```python
from build123d import *

# Parameters (mm, degrees)
BOX_W           = 42
BOX_H           = 42
BOX_DEPTH       = 5
SKETCH_R        = 2.75
POCKET_DEPTH    = 2.5
SKETCH001_R     = 1.55
POCKET001_DEPTH = 5
SKETCH002_R     = 2.75
POCKET002_DEPTH = 2.5
SKETCH003_R     = 1.55
POCKET003_DEPTH = 5
CHAMFER_SIZE    = 2
CHAMFER001_SIZE = 2
CHAMFER002_SIZE = 2
CHAMFER003_SIZE = 2
SKETCH004_W     = 16
SKETCH004_H     = 2.5
PAD_DEPTH       = 20
PAD001_DEPTH    = 2
PAD002_DEPTH    = 2
SKETCH007_R     = 1.55
POCKET004_DEPTH = 5
SKETCH008_W     = 20
SKETCH008_H     = 20
POCKET005_DEPTH = 1
SKETCH010_R     = 2.85
SKETCH010_R_2   = 1.75
POCKET006_DEPTH = 2.5
SKETCH011_R     = 1.75
SKETCH011_R_2   = 2.85
POCKET007_DEPTH = 2.5
SKETCH012_R     = 1.75
POCKET008_DEPTH = 5


with BuildPart() as part:
    # Box → Box (new body)
    with BuildSketch(Plane(origin=(-21, -21, 0), x_dir=(1, 0, 0), z_dir=(0, 0, 1))):
        with Locations((21, 21)):
            Rectangle(BOX_W, BOX_H)
    extrude(amount=BOX_DEPTH)

    # Sketch → Pocket (cut)
    with BuildSketch(Plane(origin=(-21, -21, 5), x_dir=(1, 0, 0), z_dir=(0, 0, 1))):
        with Locations((5.5, 5.5)):
            Circle(SKETCH_R)
        with Locations((36.5, 5.5)):
            Circle(SKETCH_R)
        with Locations((36.5, 36.5)):
            Circle(SKETCH_R)
        with Locations((5.5, 36.5)):
            Circle(SKETCH_R)
    extrude(amount=-POCKET_DEPTH, mode=Mode.SUBTRACT)

    # Sketch001 → Pocket001 (cut)
    with BuildSketch(Plane(origin=(-21, -21, 0), x_dir=(1, 0, 0), z_dir=(0, 0, -1))):
        with Locations((5.5, -5.5)):
            Circle(SKETCH001_R)
        with Locations((36.5, -5.5)):
            Circle(SKETCH001_R)
        with Locations((36.5, -36.5)):
            Circle(SKETCH001_R)
        with Locations((5.5, -36.5)):
            Circle(SKETCH001_R)
    extrude(amount=-POCKET001_DEPTH, mode=Mode.SUBTRACT)

    # Sketch002 → Pocket002 (cut)
    with BuildSketch(Plane(origin=(-21, -21, 0), x_dir=(1, 0, 0), z_dir=(0, 0, -1))):
        with Locations((6, -21)):
            Circle(SKETCH002_R)
        with Locations((36, -21)):
            Circle(SKETCH002_R)
    extrude(amount=-POCKET002_DEPTH, mode=Mode.SUBTRACT)

    # Sketch003 → Pocket003 (cut)
    with BuildSketch(Plane(origin=(-21, -21, 5), x_dir=(1, 0, 0), z_dir=(0, 0, 1))):
        with Locations((6, 21)):
            Circle(SKETCH003_R)
        with Locations((36, 21)):
            Circle(SKETCH003_R)
    extrude(amount=-POCKET003_DEPTH, mode=Mode.SUBTRACT)

    # Chamfer
    chamfer_edges = [part.edges().sort_by_distance(p)[0] for p in [
        (-21, -21, 2.5),
    ]]
    chamfer(chamfer_edges, length=CHAMFER_SIZE)

    # Chamfer001
    chamfer001_edges = [part.edges().sort_by_distance(p)[0] for p in [
        (-21, 21, 2.5),
    ]]
    chamfer(chamfer001_edges, length=CHAMFER001_SIZE)

    # Chamfer002
    chamfer002_edges = [part.edges().sort_by_distance(p)[0] for p in [
        (21, 21, 2.5),
    ]]
    chamfer(chamfer002_edges, length=CHAMFER002_SIZE)

    # Chamfer003
    chamfer003_edges = [part.edges().sort_by_distance(p)[0] for p in [
        (21, -21, 2.5),
    ]]
    chamfer(chamfer003_edges, length=CHAMFER003_SIZE)

    # Sketch004 → Pad (new body)
    with BuildSketch(Plane(origin=(-21, -21, 5), x_dir=(1, 0, 0), z_dir=(0, 0, 1))):
        with Locations((21, 31.25)):
            Rectangle(SKETCH004_W, SKETCH004_H)
    extrude(amount=PAD_DEPTH)

    # Sketch005 → Pad001 (new body)
    with BuildSketch(Plane(origin=(-8, -21, 0), x_dir=(0, -1, 0), z_dir=(-1, 0, 0))):
        Polygon((-30, 25), (-32.5, 25), (-41.94515, 5), (-30, 5), align=None)
    extrude(amount=PAD001_DEPTH)

    # Sketch006 → Pad002 (new body)
    with BuildSketch(Plane(origin=(8, -21, 0), x_dir=(0, 1, 0), z_dir=(1, 0, 0))):
        Polygon((30, 25), (32.5, 25), (42, 5), (30, 5), align=None)
    extrude(amount=PAD002_DEPTH)

    # Sketch007 → Pocket004 (cut)
    with BuildSketch(Plane(origin=(-21, 11.5, 0), x_dir=(-1, 0, 0), z_dir=(0, 1, 0))):
        with Locations((-21, 15)):
            Circle(SKETCH007_R)
    extrude(amount=-POCKET004_DEPTH, mode=Mode.SUBTRACT)

    # Sketch008 → Pocket005 (cut)
    with BuildSketch(Plane(origin=(-21, 9, 0), x_dir=(1, 0, 0), z_dir=(0, -1, 0))):
        with Locations((21, 15)):
            Rectangle(SKETCH008_W, SKETCH008_H)
    extrude(amount=-POCKET005_DEPTH, mode=Mode.SUBTRACT)

    # Sketch010 → Pocket006 (cut)
    with BuildSketch(Plane(origin=(-21, -21, 5), x_dir=(1, 0, 0), z_dir=(0, 0, 1))):
        with Locations((5.5, 36.5)):
            Circle(SKETCH010_R)
        with Locations((5.5, 5.5)):
            Circle(SKETCH010_R)
        with Locations((36.5, 5.5)):
            Circle(SKETCH010_R)
        with Locations((36, 21)):
            Circle(SKETCH010_R_2)
        with Locations((36.5, 36.5)):
            Circle(SKETCH010_R)
        with Locations((6, 21)):
            Circle(SKETCH010_R_2)
    extrude(amount=-POCKET006_DEPTH, mode=Mode.SUBTRACT)

    # Sketch011 → Pocket007 (cut)
    with BuildSketch(Plane(origin=(-21, -21, 0), x_dir=(1, 0, 0), z_dir=(0, 0, -1))):
        with Locations((5.5, -5.5)):
            Circle(SKETCH011_R)
        with Locations((36.5, -5.5)):
            Circle(SKETCH011_R)
        with Locations((6, -21)):
            Circle(SKETCH011_R_2)
        with Locations((36, -21)):
            Circle(SKETCH011_R_2)
        with Locations((36.5, -36.5)):
            Circle(SKETCH011_R)
        with Locations((5.5, -36.5)):
            Circle(SKETCH011_R)
    extrude(amount=-POCKET007_DEPTH, mode=Mode.SUBTRACT)

    # Sketch012 → Pocket008 (cut)
    with BuildSketch(Plane(origin=(-21, 10, 0), x_dir=(1, 0, 0), z_dir=(0, -1, 0))):
        with Locations((21, 15)):
            Circle(SKETCH012_R)
    extrude(amount=-POCKET008_DEPTH, mode=Mode.SUBTRACT)


solid = part.part
```
The model under review builds one solid part; all positions refer to its coordinate system, in mm. A direction names the side the tool comes from. Give positions to 0.01 mm unless a question says otherwise; leave off trailing zeros. Write each loop counter-clockwise with the first axis right and the second up, starting at its lowest first coordinate (ties: lowest second). Pieces come first, ordered by that corner, then holes. Notation, with made-up numbers: M 61,-35.75 L 117,-35.75 A12 ccw 117,-27.75 Z; hole C 1,-23.5 d7. An arc over 180 degrees is marked long. Write item = value, one per line. Start each with the question number.
Q1. We need section D-D (z = 7.75). State the section outline as (x, y) points.
Q2. We need section C-C (z = 15). State the section outline as (x, y) points.
Q3. Mouldability with a two-part tool opening along Y and no side actions: class faces 5 (the face through (-8.986, 16.156, 15.14)), 6 (the face through (8, 14, 11)), 7 (the face through (14, -17, 2.5)) as released by +Y, released by -Y, zero draft, split by the parting line, or undercut.
Q4. We need section B-B (x = 2.5). State the section outline as (y, z) points, plus the area to 3 significant figures.
Q5. We need section A-A (y = 0). State the section outline as (x, z) points.
Q6. For line 1 (X direction, y = 15.5, z = 0.85); line 2 (Y direction, x = -14, z = 1.25); line 3 (Y direction, x = 15.5, z = 0.8), list the stretches that pass through material, from the lowest coordinate up.
Q7. Machinability: for faces 1 (the face through (-2, 11.5, 15)), 2 (the face through (0, 10, 13)), 3 (the face through (-17, 14, 2.5)), 4 (the face through (-10, 14, 13)), which of the approach directions +Z, -Z, +X, -X, +Y, -Y give a long, thin tool a straight path to every point of the face, cutting with its end or side? Answer none if there is none.
Q8. Clearance check with flat-ended pins moving along their axes: pin 1 (10 mm diameter, centred on x = 6.5, y = -4, fed in from -Z); pin 2 (6 mm diameter, centred on x = -1.5, z = 16.5, fed in from +Y); pin 3 (4.5 mm diameter, centred on x = 15, y = 0, fed in from -Z); pin 4 (12 mm diameter, centred on x = -15, z = 13, fed in from -Y). State where each tip first meets the part, or that it passes through.
Result set:
q1.outline = M -10,10 L 10,10 L 10,19.69 L 8,19.69 L 8,11.5 L -8,11.5 L -8,19.65 L -10,19.65 Z
q2.outline = M -10,10 L -1.75,10 L -1.75,11.5 L -8,11.5 L -8,16.22 L -10,16.22 Z; M 1.75,10 L 10,10 L 10,16.25 L 8,16.25 L 8,11.5 L 1.75,11.5 Z
q3.face_5 = released by +Y
q3.face_6 = zero draft
q3.face_7 = undercut
q4.outline = M -21,0 L 21,0 L 21,5 L 11.5,5 L 11.5,25 L 10,25 L 10,5 L -21,5 Z
q4.area = 240 mm2
q5.outline = M -21,0 L -17.85,0 L -17.85,2.5 L -16.75,2.5 L -16.75,5 L -21,5 Z; M -13.25,2.5 L -12.15,2.5 L -12.15,0 L 12.15,0 L 12.15,2.5 L 13.25,2.5 L 13.25,5 L -13.25,5 Z; M 16.75,2.5 L 17.85,2.5 L 17.85,0 L 21,0 L 21,5 L 16.75,5 Z
q6.line_1 = -21 to -17.25, -13.75 to 13.75, 17.25 to 21
q6.line_2 = -21 to -16.4, -14.6 to -2.67, 2.67 to 14.6, 16.4 to 21
q6.line_3 = -21 to -17.25, -13.75 to -2.81, 2.81 to 13.75, 17.25 to 21
q7.face_1 = +Z, +Y
q7.face_2 = +Z, +X, -X, -Y
q7.face_3 = +Z
q7.face_4 = +Z, -X, +Y, -Y
q8.pin_1 = 0
q8.pin_2 = 11.5
q8.pin_3 = 2.5
q8.pin_4 = 10
